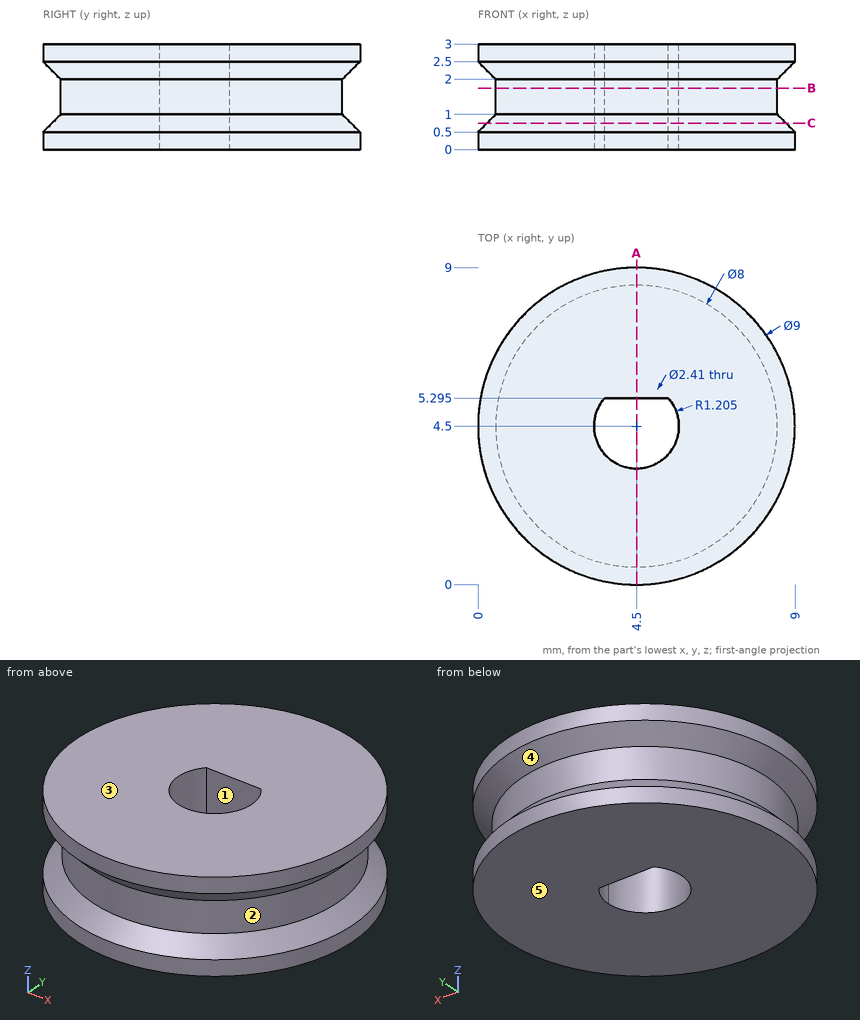
Job drawing, mm, ordinate dimensions from the low corner. One solid piece. A direction names the side the tool comes from. Round coordinates to 2 decimals unless told otherwise and drop trailing zeros. Loops run counter-clockwise (first coordinate to the right, second up) from the corner with the lowest first, then second, coordinate; pieces in that order, holes last. Notation, with made-up numbers: (74, 59) -> (105, 59) arc R22 cw to (105, 78) -> close; hole circle Ø1 at (-20.75, -21.5). An arc over 180 degrees is marked (long way). One line per item, written item: value. Start each with the question number.
Q1. Cut at A-A on x = 4.5. List the corners of the cut face in (y, z) (3 decimals).
Q2. Drop flat-ended pins along their axis: pin 1 Ø1 at (y, z) = (6, 2.5) entering from +X; pin 2 Ø0.5 at (x, z) = (4.5, 1) entering from -Y. Give the stop position or say it passes through.
Q3. Two-plate mould, pull along Z, no slides. Class the marked faces 1, 2 and 3: released by +Z, released by -Z, zero draft, split by the parting line, or undercut.
Q4. Probe line 1 along Y through (x, z) = (4.5, 1.8) (3 decimals); line 2 along X through (y, z) = (4.5, 1.35) (3 decimals); line 3 along Y through (x, z) = (4.5, 2.4) (3 decimals). List the from-to ranges inside material, lowest first.
Q5. Cut at B-B on z = 1.75. List the corners of the cut face in (x, y) (3 decimals), plus the area to 3 significant figures.
Q6. 3-axis set-ups, long thin cutter, end or side, ignore diameter. For the marked faces 4 and 5: which of +Z, -Z, +X, -X, +Y, -Y reach the whole face in a straight line?
Q7. Cut at C-C on z = 0.75. List the corners of the cut face in (x, y) (3 decimals).
Computed:
1. outline: (0, 0) -> (3.295, 0) -> (3.295, 3) -> (0, 3) -> (0, 2.5) -> (0.5, 2) -> (0.5, 1) -> (0, 0.5) -> close; (5.295, 0) -> (9, 0) -> (9, 0.5) -> (8.5, 1) -> (8.5, 2) -> (9, 2.5) -> (9, 3) -> (5.295, 3) -> close
2. pin 1: x = 8.89
2. pin 2: y = 0.25
3. face 1: zero draft
3. face 2: undercut
3. face 3: released by +Z
4. line 1: 0.5 to 3.295, 5.295 to 8.5
4. line 2: 0.5 to 3.295, 5.705 to 8.5
4. line 3: 0.1 to 3.295, 5.295 to 8.9
5. outline: circle Ø8 at (4.5, 4.5); hole (3.594, 5.295) arc R1.205 ccw (long way) to (5.406, 5.295) -> close
5. area: 46.2 mm²
6. face 4: none
6. face 5: -Z, +X, -X, +Y, -Y
7. outline: circle Ø8.5 at (4.5, 4.5); hole (3.594, 5.295) arc R1.205 ccw (long way) to (5.406, 5.295) -> close
